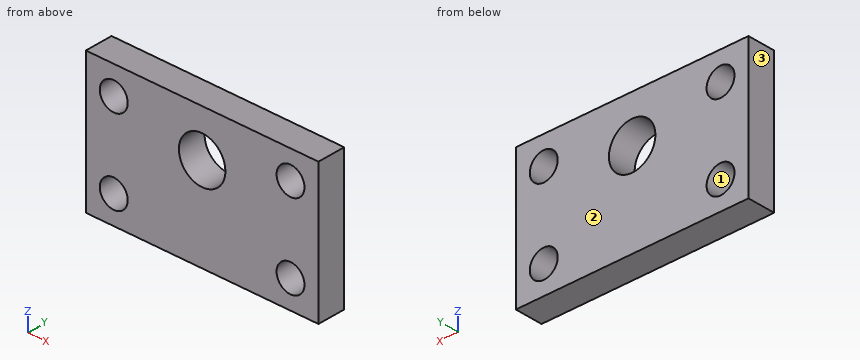
from build123d import *

# Parameters (mm, degrees)
SKETCH3_W           = 250
SKETCH3_H           = 150
BOSS_EXTRUDE2_DEPTH = 15
SKETCH5_R           = 25
CUT_EXTRUDE1_DEPTH  = 149.828760661
SKETCH6_R           = 15
CUT_EXTRUDE2_DEPTH  = 149.828760661


with BuildPart() as part:
    # Sketch3 → Boss-Extrude2 (new, symmetric)
    with BuildSketch(Plane(origin=(0, 0, 0), x_dir=(1, 0, 0), z_dir=(0, 1, 0))):
        Rectangle(SKETCH3_W, SKETCH3_H)
    extrude(amount=BOSS_EXTRUDE2_DEPTH, both=True)

    # Sketch5 → Cut-Extrude1 (cut, through all)
    with BuildSketch(Plane(origin=(0, 15, 0), x_dir=(1, 0, 0), z_dir=(0, 1, 0))):
        with Locations(Location((0, -25, 0), (0, 0, 270))):
            Circle(SKETCH5_R)
    extrude(amount=-CUT_EXTRUDE1_DEPTH, mode=Mode.SUBTRACT)

    # Sketch6 → Cut-Extrude2 (cut, through all)
    with BuildSketch(Plane(origin=(0, 15, 0), x_dir=(1, 0, 0), z_dir=(0, 1, 0))):
        with Locations(Location((-95, -45, 0), (0, 0, 270))):
            Circle(SKETCH6_R)
        with Locations(Location((95, -45, 0), (0, 0, 270))):
            Circle(SKETCH6_R)
        with Locations(Location((95, 45, 0), (0, 0, 270))):
            Circle(SKETCH6_R)
        with Locations(Location((-95, 45, 0), (0, 0, 270))):
            Circle(SKETCH6_R)
    extrude(amount=-CUT_EXTRUDE2_DEPTH, mode=Mode.SUBTRACT)


solid = part.part
CAD build for the part. Positions are in the model's coordinates, mm. Face numbers are marked on the shaded views. Coordinates: 2 decimals unless noted, no trailing zeros. Write each loop counter-clockwise with the first axis right and the second up, starting at its lowest first coordinate (ties: lowest second). Pieces come first, ordered by that corner, then holes. Notation, with made-up numbers: M 19.25,83 L 72.25,83 A30 cw 72.25,111 Z; hole C 38,11 d1. An arc over 180 degrees is marked long. Return JSON: item names as keys, results as strings.
Item 1: Slice it at A-A, the plane z = 45. Write the cut outline in (x, y).
Findings below:
{"outline": "M -125,-15 L -110,-15 L -110,15 L -125,15 Z; M -80,-15 L -15,-15 L -15,15 L -80,15 Z; M 15,-15 L 80,-15 L 80,15 L 15,15 Z; M 110,-15 L 125,-15 L 125,15 L 110,15 Z"}
Item 2: Slice it at C-C, the plane y = 5. Write the cut outline in (x, z), and give its area (3 significant figures).
Findings below:
{"outline": "M -125,-75 L 125,-75 L 125,75 L -125,75 Z; hole C -95,-45 d30; hole C -95,45 d30; hole C 0,25 d50; hole C 95,-45 d30; hole C 95,45 d30", "area": "32,700 mm2"}
Item 3: Slice it at D-D, the plane z = -45. Write the cut outline in (x, y), and give its area (3 significant figures).
Findings below:
{"outline": "M -125,-15 L -110,-15 L -110,15 L -125,15 Z; M -80,-15 L 80,-15 L 80,15 L -80,15 Z; M 110,-15 L 125,-15 L 125,15 L 110,15 Z", "area": "5,700 mm2"}
Item 4: Probe line 1 (X direction, y = 7.25, z = -45); line 2 (Z direction, x = -94, y = 12.75); line 3 (X direction, y = -1, z = 45). List the from-to ranges inside material, lowest first. Write a range as from..to.
Findings below:
{"line 1": "x = -125..-110, -80..80, 110..125", "line 2": "z = -75..-59.97, -30.03..30.03, 59.97..75", "line 3": "x = -125..-110, -80..-15, 15..80, 110..125"}
Item 5: Two-plate mould, pull along X, no slides. Class the marked faces 1, 2 and 3: +X half, -X half, draft (parallel to the pull), parting line (faces both ways), or undercut.
Findings below:
{"face 1": "undercut", "face 2": "draft", "face 3": "-X half"}
Item 6: Slice it at B-B, the plane x = -95. Write the cut outline in (y, z).
Findings below:
{"outline": "M -15,-75 L 15,-75 L 15,-60 L -15,-60 Z; M -15,-30 L 15,-30 L 15,30 L -15,30 Z; M -15,60 L 15,60 L 15,75 L -15,75 Z"}
